Check sheet for the modelled part. Datum: model origin and axes. Units: mm. Face numbers are marked on the shaded views. A direction names the side the tool comes from. Coordinates: 2 decimals unless noted, no trailing zeros. Loops run counter-clockwise (first coordinate to the right, second up) from the corner with the lowest first, then second, coordinate; pieces in that order, holes last. Notation, with made-up numbers: (61, 10) -> (93, 10) arc R10 ccw to (93, 19) -> close; hole circle Ø9 at (76.25, 13). An arc over 180 degrees is marked (long way). Use CSV: the item, a comma, the result in double quotes. Start each with the question number.
1. Sectioned sample at B-B, the plane y = 8. Record the cut outline in (x, z), and give its area (3 significant figures).
2. Release check for a two-part mould opening along Z. For the marked faces 1, 2, 3 and 4 record: pulls with the +Z half, pulls with the -Z half, needs draft (parallel to the pull), parting line crosses it, or undercut.
3. Gauge pin test, flat ends, axial feed: pin 1 (1.5 mm diameter, centred on x = 15, z = -46, fed in from +Y); pin 2 (2 mm diameter, centred on x = 80, y = 32, fed in from -Z); pin 3 (1.6 mm diameter, centred on x = 75, y = 35.5, fed in from -Z). Record the tip position at first contact, or that the pin passes through.
4. Sectioned sample at C-C, the plane y = 19. Record the cut outline in (x, z), and give its area (3 significant figures).
5. Sectioned sample at A-A, the plane z = -18.5. Record the cut outline in (x, y).
6. Thickness scan on L1, parallel to Z at x = 63, y = 20; L2, parallel to Z at x = 70.5, y = 19.5; L3, parallel to Y at x = 60, z = -17. Record the ranges inside material, lowest first.
7. Set-up check for the marked faces 5, 6, 7, 8 and 9: record each of +Z, -Z, +X, -X, +Y, -Y from which the full face is reachable in a straight line by a thin tool's end or side.
```python
from build123d import *

# Parameters (mm, degrees)
F1_DEPTH = 100
F2_R     = 2


with BuildPart() as f1:
    # F0 (on Right) → F1 (new body)
    with BuildSketch(Plane.YZ):
        Polygon((34, -23), (36, -23), (36, 0), (0, 0), (0, -96), (27, -96), (27, -81), (14.755062, -66.407052), (27.642788, -51.048059), (27.642788, -41.048059), (25.642788, -41.048059), (25.642788, -50.320118), (12.144248, -66.407052), (25, -81.72794), (25, -94), (2, -94), (2, -2), (34, -2), align=None)
    extrude(amount=F1_DEPTH)

    # F2
    f2_edges = [f1.edges().sort_by_distance(p)[0] for p in [
        (50, 36, 0),
        (50, 0, 0),
        (50, 34, -2),
        (50, 2, -2),
        (50, 0, -96),
        (50, 27, -96),
        (50, 27, -81),
        (50, 14.755062, -66.407052),
        (50, 27.642788, -51.048059),
        (50, 2, -94),
        (50, 25, -94),
        (50, 25, -81.72794),
        (50, 12.144248, -66.407052),
        (50, 25.642788, -50.320118),
    ]]
    fillet(f2_edges, radius=F2_R)


solid = f1.part
```
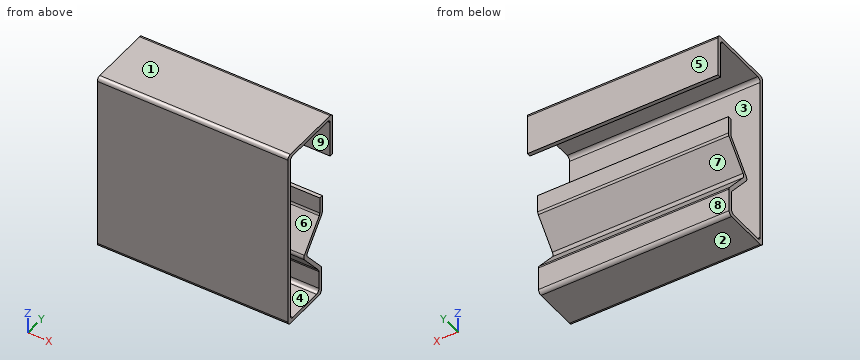
Completed:
1,outline,"(0, -96) -> (100, -96) -> (100, -94) -> (0, -94) -> close; (0, -2) -> (100, -2) -> (100, 0) -> (0, 0) -> close"
1,area,"400 mm²"
2,face 1,"pulls with the +Z half"
2,face 2,"pulls with the -Z half"
2,face 3,"undercut"
2,face 4,"undercut"
3,pin 1,"y = 27.64"
3,pin 2,"z = -2.27"
3,pin 3,"z = -23"
4,outline,"(0, -96) -> (100, -96) -> (100, -94) -> (0, -94) -> close; (0, -74.58) -> (100, -74.58) -> (100, -71.47) -> (0, -71.47) -> close; (0, -61.35) -> (100, -61.35) -> (100, -58.24) -> (0, -58.24) -> close; (0, -2) -> (100, -2) -> (100, 0) -> (0, 0) -> close"
4,area,"1,020 mm²"
5,outline,"(0, 0) -> (100, 0) -> (100, 2) -> (0, 2) -> close; (0, 34) -> (100, 34) -> (100, 36) -> (0, 36) -> close"
6,L1,"-96 to -94, -75.77 to -72.66, -60.16 to -57.04, -2 to 0"
6,L2,"-96 to -94, -75.17 to -72.06, -60.75 to -57.64, -2 to 0"
6,L3,"0 to 2, 34 to 36"
7,face 5,"+Z, -Z, +X, -X, +Y"
7,face 6,"+X, -X"
7,face 7,"+X, -X, +Y"
7,face 8,"-Z, +X, -X, +Y"
7,face 9,"-Z, +X, -X"
